from build123d import *

# Parameters (mm, degrees)
SCHIZZO1_R             = 10
ESTRUSIONE1_DEPTH      = 4
SCHIZZO2_W             = 4
SCHIZZO2_H             = 20
ESTRUSIONE2_DEPTH      = 226
RIPETIZIONE_A_L1_COUNT = 2
RIPETIZIONE_A_L1_PITCH = 222
RACCORDO1_R            = 5
RACCORDO2_R            = 2


with BuildPart() as part:
    # Schizzo1 → Estrusione1 (new body)
    with BuildSketch(Plane.XY):
        with BuildLine():
            Line((-26, 0), (-11.115384615, 12.862667875))
            ThreePointArc((-11.115384615, 12.862667875), (15.70846037, 6.499559431), (1.222434951, -16.955991649))
            Line((1.222434951, -16.955991649), (-41, -20))
            Line((-41, -20), (-45, -20))
            Line((-45, -20), (-45, 0))
            Line((-45, 0), (-26, 0))
        make_face()
        Circle(SCHIZZO1_R, mode=Mode.SUBTRACT)
    estrusione1 = extrude(amount=ESTRUSIONE1_DEPTH)

    # Schizzo2 → Estrusione2 (add)
    with BuildSketch(Plane.XY.offset(4)):
        with Locations((-43, -10)):
            Rectangle(SCHIZZO2_W, SCHIZZO2_H)
    extrude(amount=-ESTRUSIONE2_DEPTH)

    # Ripetizione a L1: Estrusione1 ×2
    with Locations(*[(0, 0, -i * RIPETIZIONE_A_L1_PITCH) for i in range(1, RIPETIZIONE_A_L1_COUNT)]):
        add(estrusione1)

    # Raccordo1
    raccordo1_edges = [part.edges().sort_by_distance(p)[0] for p in [
        (-45, -10, -222),
        (-45, -10, 4),
    ]]
    fillet(raccordo1_edges, radius=RACCORDO1_R)

    # Raccordo2
    raccordo2_edges = [part.edges().sort_by_distance(p)[0] for p in [
        (-41, -10, 0),
        (-41, -10, -218),
    ]]
    fillet(raccordo2_edges, radius=RACCORDO2_R)


solid = part.part
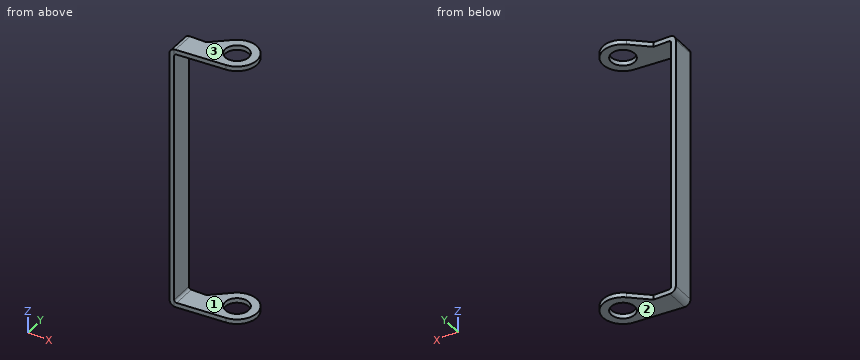
The listing builds one solid part. Answer for the finished solid, in the listing's coordinates (mm). Face numbers are marked on the shaded views. Round coordinates to 2 decimals unless told otherwise and drop trailing zeros. Write each loop counter-clockwise with the first axis right and the second up, starting at its lowest first coordinate (ties: lowest second). Pieces come first, ordered by that corner, then holes. Notation, with made-up numbers: M -34.5,-30 L 17.5,-30 A11 ccw 17.5,-12 Z; hole C 29,41.25 d2. An arc over 180 degrees is marked long. Write each question's results on one line, items separated by ' | '. Start each with the question number.
Item 1: A cutting plane is placed at C-C on x = -3. Write down the section's boundary in (y, z), and give its area (3 significant figures).
Item 2: For a pull along Z with two mould halves and no side action, classify the marked faces 1, 2 and 3 as pulls with the +Z half, pulls with the -Z half, needs draft (parallel to the pull), parting line crosses it, or undercut.
Item 3: A cutting plane is placed at B-B on x = -34. Write down the section's boundary in (y, z), and give its area (3 significant figures).
Item 4: A cutting plane is placed at A-A on y = 2.5. Write down the section's boundary in (x, z).
Item 5: A cutting plane is placed at D-D on z = -117. Write down the section's boundary in (x, y).
Item 6: Straight lines are drawn through the part: L1, parallel to Z at x = 2.5, y = 13; L2, parallel to X at y = -8.5, z = -183.5; L3, parallel to Y at x = -41.5, z = -92. For each, find the intervals that lie inside material, in ascending order. Write a range as [from, to].
Item 7: Flat-ended cylindrical pins translate along their axes: pin 1 Ø12 at (x, y) = (0, 0) entering from +Z; pin 2 Ø16 at (y, z) = (-13, -147) entering from +X. Find the tip coordinate at first contact, or state that the pin passes through.
Check sheet entries:
1) outline: M -17.26,-222 L -9.54,-222 L -9.54,-218 L -17.26,-218 Z; M -17.26,0 L -9.54,0 L -9.54,4 L -17.26,4 Z; M 9.54,-222 L 16.73,-222 L 16.73,-218 L 9.54,-218 Z; M 9.54,0 L 16.73,0 L 16.73,4 L 9.54,4 Z | area: 119 mm²
2) face 1: undercut | face 2: pulls with the -Z half | face 3: pulls with the +Z half
3) outline: M -19.5,-222 L 0,-222 L 0,-218 L -19.5,-218 Z; M -19.5,0 L 0,0 L 0,4 L -19.5,4 Z | area: 156 mm²
4) outline: M -23.11,-222 L -9.68,-222 L -9.68,-218 L -23.11,-218 Z; M -23.11,0 L -9.68,0 L -9.68,4 L -23.11,4 Z; M 9.68,-222 L 16.82,-222 L 16.82,-218 L 9.68,-218 Z; M 9.68,0 L 16.82,0 L 16.82,4 L 9.68,4 Z
5) outline: M -45,-20 L -41,-20 L -41,0 L -45,0 Z
6) L1: [-222, -218], [0, 4] | L2: [-45, -41] | L3: [-20, 0]
7) pin 1: through | pin 2: x = -41
